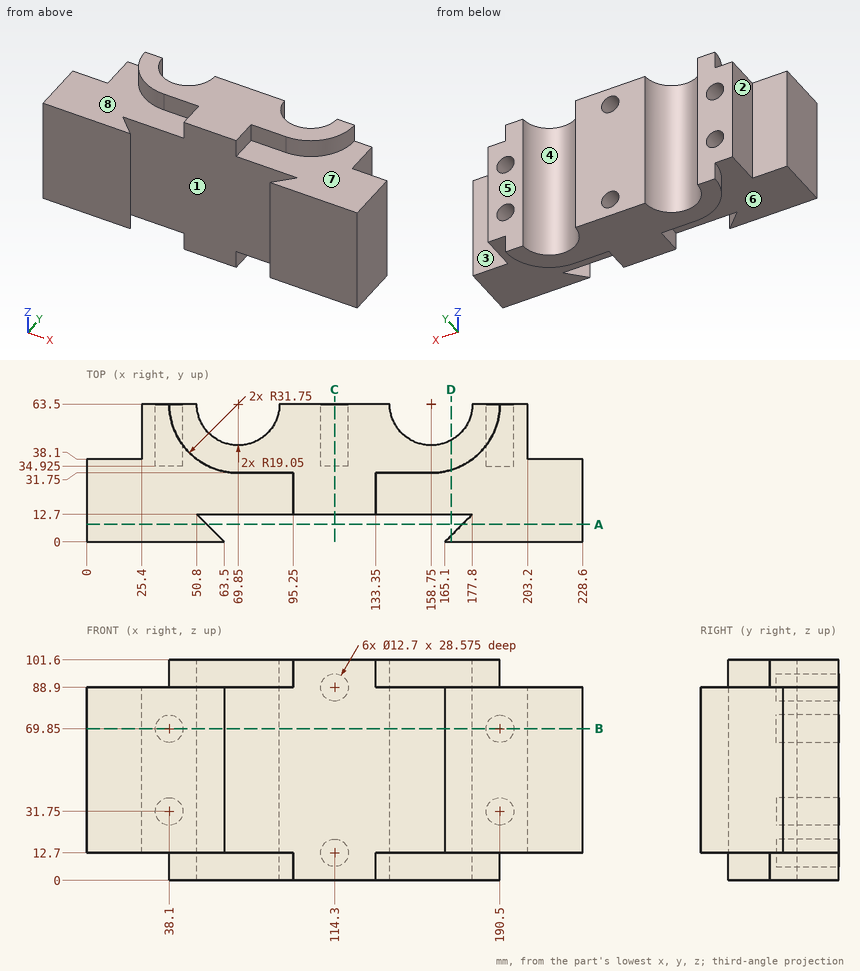
Answer from the drawing. Dimensions are ordinates in mm from the lowest x, y and z of the part. A direction names the side the tool comes from. Round coordinates to 2 decimals unless told otherwise and drop trailing zeros. Write each loop counter-clockwise with the first axis right and the second up, starting at its lowest first coordinate (ties: lowest second). Pieces come first, ordered by that corner, then holes. Notation, with made-up numbers: (61.25, 58.25) - (117.25, 58.25) arc R17 ccw to (117.25, 80.25) - close; hole circle Ø8 at (67.5, 65.5). An arc over 180 degrees is marked (long way). One line per item, written item: value.
Q1. Find section B-B (z = 69.85). Determine the outline of the cut face in (x, y) (3 decimals), and give its area (3 significant figures).
The answers:
outline: (0, 0) - (63.5, 0) - (50.8, 12.7) - (177.8, 12.7) - (165.1, 0) - (228.6, 0) - (228.6, 38.1) - (203.2, 38.1) - (203.2, 63.5) - (196.85, 63.5) - (196.85, 34.925) - (184.15, 34.925) - (184.15, 63.5) - (177.8, 63.5) arc R19.05 cw to (139.7, 63.5) - (88.9, 63.5) arc R19.05 cw to (50.8, 63.5) - (44.45, 63.5) - (44.45, 34.925) - (31.75, 34.925) - (31.75, 63.5) - (25.4, 63.5) - (25.4, 38.1) - (0, 38.1) - close
area: 9,910 mm2
Q2. Find section C-C (x = 114.3). Determine the outline of the cut face in (y, z) (3 decimals).
The answers:
outline: (12.7, 0) - (63.5, 0) - (63.5, 6.35) - (34.925, 6.35) - (34.925, 19.05) - (63.5, 19.05) - (63.5, 82.55) - (34.925, 82.55) - (34.925, 95.25) - (63.5, 95.25) - (63.5, 101.6) - (12.7, 101.6) - close
Q3. For a pull along X with two mould halves and no side action, classify the marked faces 1, 2, 3 and 4 as pulls with the +X half, pulls with the -X half, needs draft (parallel to the pull), parting line crosses it, or undercut.
The answers:
face 1: undercut
face 2: pulls with the -X half
face 3: needs draft
face 4: undercut
Q4. Find section A-A (y = 8). Determine the outline of the cut face in (x, z).
The answers:
outline: (0, 12.7) - (55.5, 12.7) - (55.5, 88.9) - (0, 88.9) - close; (173.1, 12.7) - (228.6, 12.7) - (228.6, 88.9) - (173.1, 88.9) - close
Q5. Straight lines are drawn through the part: line 1 (X direction, y = 40, z = 31); line 2 (X direction, y = 51, z = 88.5); line 3 (X direction, y = 53, z = 86). For each, find the intervals that lie inside material, in ascending order. Write a range as from..to.
The answers:
line 1: x = 25.4..31.79, 44.41..184.19, 196.81..203.2
line 2: x = 25.4..55.47, 84.23..107.96, 120.64..144.37, 173.13..203.2
line 3: x = 25.4..53.95, 85.75..108.65, 119.95..142.85, 174.65..203.2
Q6. Find section D-D (x = 168). Determine the outline of the cut face in (y, z), and give its area (3 significant figures).
The answers:
outline: (0, 12.7) - (2.9, 12.7) - (2.9, 88.9) - (0, 88.9) - close; (12.7, 12.7) - (33.13, 12.7) - (33.13, 0) - (46.85, 0) - (46.85, 101.6) - (33.13, 101.6) - (33.13, 88.9) - (12.7, 88.9) - close
area: 3,170 mm2
Q7. Each of these flat-tipped pins is pushed along its axis until it touches: P1, Ø1, axis at x = 145.5, z = 54, coming from the +Y side; P2, Ø2, axis at x = 190.5, y = 40.5, coming from the +Z side; P3, Ø20.5, axis at y = 54.5, z = 63, coming from the -X side; P4, Ø8, axis at y = 25.5, z = 74.5, coming from the -X side. Where does it stop, or does it pass through?
The answers:
P1: stops at y = 50.32
P2: stops at z = 88.9
P3: stops at x = 25.4
P4: stops at x = 0
Q8. Which of the six approach directions +Z, -Z, +X, -X, +Y, -Y give full straight-line access (tool end or side, diameter ignored) to the marked faces 5, 6, 7 and 8?
The answers:
face 5: +Z, -Z, +X, -X, +Y
face 6: -Z, -X, -Y
face 7: +Z, +X, -Y
face 8: +Z, -X, -Y
